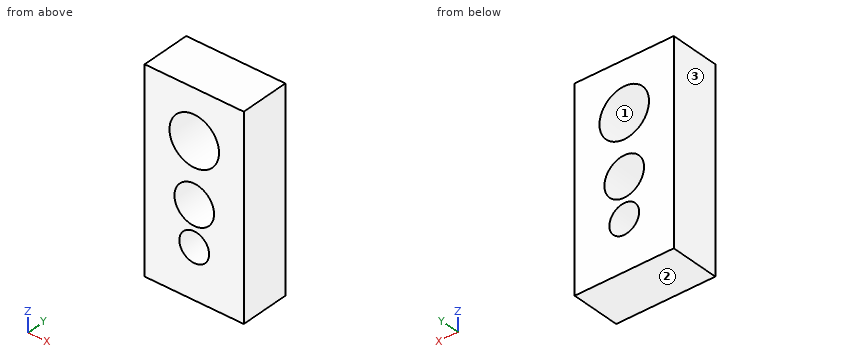
from build123d import *

# Parameters (mm, degrees)
F0_W     = 20
F0_H     = 40
F0_R     = 3
F0_R_2   = 4
F0_R_3   = 5
F1_DEPTH = 10


with BuildPart() as f1:
    # F0 (on Front) → F1 (new body)
    with BuildSketch(Plane.XZ):
        with Locations((0, 10)):
            Rectangle(F0_W, F0_H)
        Circle(F0_R, mode=Mode.SUBTRACT)
        with Locations((0, 8)):
            Circle(F0_R_2, mode=Mode.SUBTRACT)
        with Locations((0, 20)):
            Circle(F0_R_3, mode=Mode.SUBTRACT)
    extrude(amount=F1_DEPTH)


solid = f1.part
Verification items for the finished model (mm, model axes). Face numbers are marked on the shaded views. Coordinates: 2 decimals unless noted, no trailing zeros. Order: outer loops, then holes, each group sorted by start corner. A loop starts at its lowest first (then second) coordinate and runs counter-clockwise, first axis right, second up.
1. Sectioned sample at A-A, the plane x = 0. Record the cut outline in (y, z).
Results found:
outline: (-10, -10) - (0, -10) - (0, -3) - (-10, -3) - close; (-10, 3) - (0, 3) - (0, 4) - (-10, 4) - close; (-10, 12) - (0, 12) - (0, 15) - (-10, 15) - close; (-10, 25) - (0, 25) - (0, 30) - (-10, 30) - close
2. Scan lines: line 1 (Z direction, x = 0, y = -2.5); line 2 (X direction, y = -1.5, z = 5); line 3 (X direction, y = -2.75, z = 18.5). Record each from-to range of solid material in increasing order.
Results found:
line 1: z = -10 to -3, 3 to 4, 12 to 15, 25 to 30
line 2: x = -10 to -2.65, 2.65 to 10
line 3: x = -10 to -4.77, 4.77 to 10
3. Sectioned sample at C-C, the plane y = -4.5. Record the cut outline in (x, z), and give its area (3 significant figures).
Results found:
outline: (-10, -10) - (10, -10) - (10, 30) - (-10, 30) - close; hole circle Ø10 at (0, 20); hole circle Ø8 at (0, 8); hole circle Ø6 at (0, 0)
area: 643 mm2
4. Sectioned sample at B-B, the plane z = 20. Record the cut outline in (x, y).
Results found:
outline: (-10, -10) - (-5, -10) - (-5, 0) - (-10, 0) - close; (5, -10) - (10, -10) - (10, 0) - (5, 0) - close
5. Sectioned sample at D-D, the plane z = 8. Record the cut outline in (x, y).
Results found:
outline: (-10, -10) - (-4, -10) - (-4, 0) - (-10, 0) - close; (4, -10) - (10, -10) - (10, 0) - (4, 0) - close
6. Release check for a two-part mould opening along Z. For the marked faces 1, 2 and 3 record: +Z half, -Z half, draft (parallel to the pull), parting line (faces both ways), or undercut.
Results found:
face 1: undercut
face 2: -Z half
face 3: draft
